Autodesk Inventor part; units mm, degrees
ref_plane "YZ Plane" through (0, 0, 0) normal (1, 0, 0) x (0, 1, 0)
ref_plane "XZ Plane" through (0, 0, 0) normal (0, 1, 0) x (-1, 0, 0)
ref_plane "XY Plane" through (0, 0, 0) normal (0, 0, 1) x (1, 0, 0)
sketch "Boceto1" plane through (0, 0, 0) normal (0, 0, 1) x (1, 0, 0)
  line L0 (-32, 50.5) -> (-32, 23)
  line L1 (-32, 23) -> (-30, 8)
  line L2 (-30, 8) -> (-30, 0)
  line L3 (-32, 50.5) -> (-28.5, 50.5)
  line L4 (-24, 23.6746) -> (-21.5, 23.6746)
  line L5 (-21.5, 23.6746) -> (-27, 0)
  line L6 (-27, 0) -> (-30, 0)
  line L7 (-28.5, 50.5) -> (-24, 23.6746)
  line L8 (0, -10.1) -> (0, 60.6)
  point P0 (0, 0)
  point P1 (0, 0)
  dimension "d2" = 2
  dimension "d3" = 8
  dimension "d4" = 15
  dimension "d14" = 3.5
  dimension "d15" = 3
  dimension "d16" = 2.5
  dimension "d17" = 4.5
revolve "Revolución1" add sketch "Boceto1" angle 360 about axis through (0, -10, 0) along (0, 1, 0)
properties part number "PARTE_INTERIOR_FENOLICO_TOBERA" material "Resina fenólica"
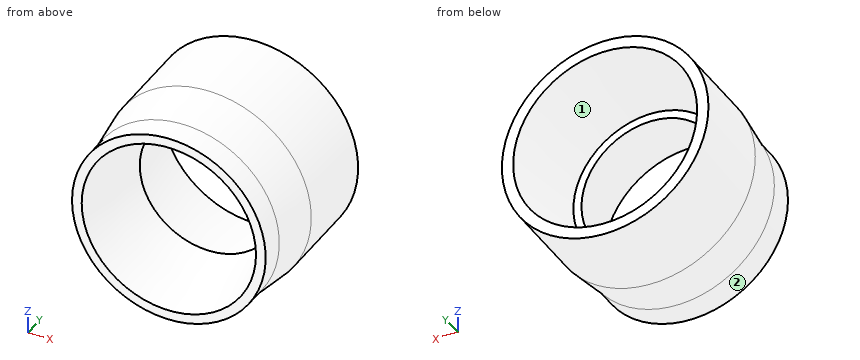
Build history of the part. All positions in model axes, mm. Face numbers are marked on the shaded views. Round coordinates to 2 decimals unless told otherwise and drop trailing zeros. Order: outer loops, then holes, each group sorted by start corner. A loop starts at its lowest first (then second) coordinate and runs counter-clockwise, first axis right, second up. Notation, with made-up numbers: (-3.75, -13) -> (44.25, -13) arc R23 cw to (44.25, 3) -> close; hole circle Ø10 at (44, 19). An arc over 180 degrees is marked (long way). Answer in a Markdown table with one row per item.
1) Mould opens along X. For the marked faces 1 and 2 say: released by +X, released by -X, zero draft, split by the parting line, or undercut.
Values:
| item | result |
|---|---|
| face 1 | undercut |
| face 2 | split by the parting line |
2) Band-saw the part on A-A on x = 0. Give the cut face in (y, z).
Values:
| item | result |
|---|---|
| outline | (0, -30) -> (8, -30) -> (23, -32) -> (50.5, -32) -> (50.5, -28.5) -> (23.67, -24) -> (23.67, -21.5) -> (0, -27) -> close; (0, 27) -> (23.67, 21.5) -> (23.67, 24) -> (50.5, 28.5) -> (50.5, 32) -> (23, 32) -> (8, 30) -> (0, 30) -> close |
3) Band-saw the part on C-C on y = 17.5. Give the cut face in (x, z), and give its area (3 significant figures).
Values:
| item | result |
|---|---|
| outline | circle Ø62.53 at (0, 0); hole circle Ø45.87 at (0, 0) |
| area | 1,420 mm2 |
4) Pin check, flat tips, straight feed: P1, Ø4, axis at x = -16.5, y = 44.5, coming from the -Z side; P2, Ø24, axis at x = -1.5, z = 4.5, coming from the +Y side; P3, Ø10, axis at y = 39.5, z = -6.5, coming from the -X side; P4, Ø10, axis at x = -2.5, y = 38.5, coming from the +Z side. Stop position of each tip, or through.
Values:
| item | result |
|---|---|
| P1 | z = -28.53 |
| P2 | through |
| P3 | x = -31.96 |
| P4 | z = 32 |
5) Wall check: L1, parallel to X at y = 44, z = 8.5; L2, parallel to Z at x = 15.5, y = 15; L3, parallel to Z at x = 4, y = 22. Give the ranges that are in metal, low to high.
Values:
| item | result |
|---|---|
| L1 | -30.85 to -26.06, 26.06 to 30.85 |
| L2 | -26.77 to -17.68, 17.68 to 26.77 |
| L3 | -31.61 to -21.52, 21.52 to 31.61 |
6) Band-saw the part on D-D on y = 32. Give the cut face in (x, z), and give its area (3 significant figures).
Values:
| item | result |
|---|---|
| outline | circle Ø64 at (0, 0); hole circle Ø50.79 at (0, 0) |
| area | 1,190 mm2 |
7) Band-saw the part on B-B on z = 0. Give the cut face in (x, y).
Values:
| item | result |
|---|---|
| outline | (-32, 23) -> (-30, 8) -> (-30, 0) -> (-27, 0) -> (-21.5, 23.67) -> (-24, 23.67) -> (-28.5, 50.5) -> (-32, 50.5) -> close; (21.5, 23.67) -> (27, 0) -> (30, 0) -> (30, 8) -> (32, 23) -> (32, 50.5) -> (28.5, 50.5) -> (24, 23.67) -> close |
